Here's how the part is built. I have some questions about the finished solid (model axes, mm). A direction names the side the tool comes from. Give positions to 0.01 mm unless a question says otherwise; leave off trailing zeros. Write each loop counter-clockwise with the first axis right and the second up, starting at its lowest first coordinate (ties: lowest second). Pieces come first, ordered by that corner, then holes. Notation, with made-up numbers: (13, 85.25) -> (56, 85.25) arc R5 ccw to (56, 93.25) -> close; hole circle Ø8 at (51, 48). An arc over 180 degrees is marked (long way). Answer as CSV lines item,"result". Start each with the question number.
Autodesk Inventor part; units mm, degrees
ref_plane "Work Plane1" through (1.525, 0, 0) normal (0, 0, 1) x (1, 0, 0)
ref_plane "YZ Plane" through (0, 0, 0) normal (1, 0, 0) x (0, 1, 0)
ref_plane "XZ Plane" through (0, 0, 0) normal (0, 1, 0) x (-1, 0, 0)
sketch "Sketch1" plane through (0, 0, 0) normal (0, 0, 1) x (1, 0, 0)
  line L0 (0, 4) -> (40, 4)
  line L1 (40, 4) -> (40, 0)
  line L2 (40, 0) -> (0, 0)
  line L3 (-8, 0) -> (48, 0)
  line L4 (0, -0.8) -> (0, 4.8)
  line L5 (0, 4) -> (0, 0)
  dimension "d2" = 8
  dimension "d59" = 40
revolve "Body" add sketch "Sketch1" angle 360 about axis through (40, 0, 0) along (-1, 0, 0)
sketch "Sketch2" plane through (0, 0, 0) normal (-1, 0, 0) x (0, 0, 1)
  line L0 (0, 7.5056) -> (6.5, 3.7528)
  line L1 (6.5, 3.7528) -> (6.5, -3.7528)
  line L2 (6.5, -3.7528) -> (0, -7.5056)
  line L3 (0, -7.5056) -> (-6.5, -3.7528)
  line L4 (-6.5, -3.7528) -> (-6.5, 3.7528)
  line L5 (-6.5, 3.7528) -> (0, 7.5056)
  line L6 (-9.1, 0) -> (9.1, 0)
  line L7 (0, 10.5078) -> (0, -10.5078)
  point P0 (0, 0)
  point P1 (0, 0)
  dimension "d11" = 13
extrude "Head" add sketch "Sketch2" along normal blind 5.68
sketch "Sketch4" plane through (0, 0, 0) normal (0, 0, 1) x (1, 0, 0)
  line L0 (-4.9294, 7.8) -> (-5.68, 6.5)
  line L1 (-1.1, 0) -> (-0.234, 0)
  line L2 (-6.7692, 0) -> (0.8552, 0)
  line L3 (-5.68, 7.8) -> (-4.9294, 7.8)
  line L4 (-5.68, 6.5) -> (-5.68, 7.8)
  line L5 (0, 9.36) -> (0, -1.56)
  dimension "d65" = 13
  dimension "d67" = 30
  dimension "d68" = 15.6
  dimension "d69" = 5.68
revolve "Chamfer1" cut sketch "Sketch4" angle 360 about axis through (-1.1, 0, 0) along (1, 0, 0)
thread "Thread"
chamfer "Chamfer2" distance 0.7668 distance2 0.7669 1 edges at (40, -4, 0) measured on face at (40, 0.4453, 1.0204)
fillet "Fillet" radius 0.1 1 edges at (0, -4, 0)
ref_plane "Work Plane1" through (1.525, 0, 0) normal (0, 0, 1) x (1, 0, 0)
equation "\"d2\" = GD"
equation "\"d59\" = NLG"
equation "\"d11\" = SW"
equation "\"d3\" = KOH"
equation "\"d15\" = GEL"
equation "\"d6\" = -0.5 * SPD + 0.5 * GD"
equation "\"d71\" = RR"
equation "\"d65\" = SW"
equation "\"d67\" = ANG1"
equation "\"d68\" = 1.2 * SW"
equation "\"d69\" = KOH"
equation "\"NLG\" = 40"
equation "\"GD\" = NND"
equation "\"BDM\" = NND"
equation "\"KOH\" = 5.68"
equation "\"GEL\" = 22"
equation "\"SW\" = 13"
equation "\"SW0\" = SW"
equation "\"SPD\" = NND - 1.2269 * PTC"
equation "\"SD2\" = NND"
equation "\"SD\" = 0"
equation "\"ANG1\" = 30deg"
equation "\"GAL\" = 0.61345 * PTC"
equation "\"GUL\" = 0.61345 * PTC"
equation "\"RR\" = 0.1"
equation "\"RR1\" = 0.4"
equation "\"GD1\" = THREADDIA - 1.2269 * PTC"
equation "\"THREADDIA\" = 8"
equation "\"TOA\" = 30deg"
equation "\"PTC\" = 1.25"
equation "\"KOH1\" = 3.7"
equation "\"NND\" = 8"
equation "\"E0\" = 1.155 * SW"
properties part number "ANSI B18.2.3.5M - M8 x 1.25 x 40" material "Steel, Mild"
Item 1: If we section it at A-A (x = -0.5): Please give me the cut outline in (y, z).
Item 2: I'm going to push flat-ended pins straight in: pin 1 (2 mm diameter, centred on x = 9, z = 1.5, fed in from -Y); pin 2 (6 mm diameter, centred on x = 28, z = -4.5, fed in from -Y); pin 3 (3 mm diameter, centred on x = 3.5, z = 1.5, fed in from +Y). Where does each tip first touch, or does it pass through?
Item 3: For faces 1 (the face through (19.94, -0.867, -3.905)), 2 (the face through (-2.8, 5.66, 3.2)), which set-ups out of +Z, -Z, +X, -X, +Y, -Y let a thin tool reach every point of the face, with its end or its side?
Item 4: If we section it at B-B (x = 25.5): Please give me the cut outline in (y, z), and give its area (3 significant figures).
Item 5: If I drill on line 1 (X direction, y = 1.25, z = 4.25); line 2 (Y direction, x = 12.5, z = -2.5); line 3 (Y direction, x = 19, z = -1), over which ranges is the centre line in solid material (lowest first)? Write a range as [from, to].
Final values:
1,outline,"(-7.51, 0) -> (-3.75, -6.5) -> (3.75, -6.5) -> (7.51, 0) -> (3.75, 6.5) -> (-3.75, 6.5) -> close"
2,pin 1,"y = -3.97"
2,pin 2,"y = -3.71"
2,pin 3,"y = 4"
3,face 1,"+X"
3,face 2,"+Z, +X, -X, +Y"
4,outline,"circle Ø8 at (0, 0)"
4,area,"50.3 mm2"
5,line 1,"[-5.68, 0]"
5,line 2,"[-3.12, 3.12]"
5,line 3,"[-3.87, 3.87]"
